Build history of the part. All positions in model axes, mm. Face numbers are marked on the shaded views. A direction names the side the tool comes from. Give positions to 0.01 mm unless a question says otherwise; leave off trailing zeros. Loops run counter-clockwise (first coordinate to the right, second up) from the corner with the lowest first, then second, coordinate; pieces in that order, holes last. Notation, with made-up numbers: (-5.75, -19.75) -> (29.25, -19.75) arc R16 ccw to (29.25, -3.75) -> close; hole circle Ø7 at (34, 81). An arc over 180 degrees is marked (long way). Answer as a JSON object with one key per item and string values. Group by question number.
Q1. Wall check: probe 1 along Y at (x, z) = (15, -64.5); probe 2 along Y at (x, z) = (-15, -63); probe 3 along X at (y, z) = (1.5, 23.5). Give the ranges that are in metal, low to high. Write a range as from..to.
Q2. Band-saw the part on C-C, the plane z = 39. Write the cut outline in (x, y), plus the area to 3 significant figures.
Q3. Tool access for the marked faces 4, 5, 6, 7 and 8: list every direction of +Z, -Z, +X, -X, +Y, -Y with a clear straight run to the whole face (end or side of a thin tool).
Q4. Drop flat-ended pins along their axis: pin 1 (4 mm diameter, centred on y = -21.5, z = 9, fed in from -X); pin 2 (3 mm diameter, centred on x = 11, z = -66.5, fed in from -Y); pin 3 (10 mm diameter, centred on x = 24, y = -38, fed in from -Z). Give the stop position or say it passes through.
Q5. Band-saw the part on D-D, the plane x = -20.5. Write the cut outline in (y, z).
Q6. Band-saw the part on B-B, the plane x = 18. Write the cut outline in (y, z), plus the area to 3 significant figures.
Q7. Band-saw the part on A-A, the plane x = -8. Write the cut outline in (y, z).
Q8. Two-plate mould, pull along Z, no slides. Class the marked faces 1, 2 and 3: pulls with the +Z half, pulls with the -Z half, needs draft (parallel to the pull), parting line crosses it, or undercut.
from build123d import *

# Parameters (mm, degrees)
SKETCH1_R                     = 25
BOSS_EXTRUDE1_DEPTH           = 75
SKETCH2_R                     = 19
BOSS_EXTRUDE2_DEPTH           = 31.75
BOSS_EXTRUDE2_TAPER           = 3
BOSS_EXTRUDE2_OTHER_WAY_DEPTH = 31.75
BOSS_EXTRUDE2_OTHER_WAY_TAPER = 3
CUT_EXTRUDE2_DEPTH            = 161.296002109
CUT_EXTRUDE3_DEPTH            = 161.296002109
SKETCH14_R                    = 12.5
CUT_EXTRUDE4_DEPTH            = 149.240724994
SKETCH16_R                    = 8
CUT_EXTRUDE5_DEPTH            = 159.112302029


with BuildPart() as part:
    # Sketch1 → Boss-Extrude1 (new body)
    with BuildSketch(Plane.XY):
        Circle(SKETCH1_R)
    extrude(amount=BOSS_EXTRUDE1_DEPTH)



with BuildPart() as body_2:
    # Sketch2 → Boss-Extrude2 (new body)
    with BuildSketch(Plane(origin=(0, 0, 0), x_dir=(0, 0, -1), z_dir=(1, 0, 0))):
        with Locations((63.5, -100)):
            Circle(SKETCH2_R)
    extrude(amount=BOSS_EXTRUDE2_DEPTH, taper=BOSS_EXTRUDE2_TAPER)

    # Sketch2 → Boss-Extrude2 other way (add)
    with BuildSketch(Plane(origin=(0, 0, 0), x_dir=(0, 0, -1), z_dir=(1, 0, 0))):
        with Locations((63.5, -100)):
            Circle(SKETCH2_R)
    extrude(amount=-BOSS_EXTRUDE2_OTHER_WAY_DEPTH, taper=BOSS_EXTRUDE2_OTHER_WAY_TAPER)


with BuildPart() as part_1:
    add(part.part)

    add(body_2.part)  # Sweep2 merges body 2
    # Sweep2: sweep along a path in Sketch5
    with BuildLine(Plane(origin=(0, 0, 0), x_dir=(0, 0, -1), z_dir=(1, 0, 0))) as sweep2_path:
        Line((63.5, -81), (8, -81))
        ThreePointArc((8, -81), (-6.142135624, -75.142135624), (-12, -61))
        Line((-12, -61), (-12, 0))
    # Sketch6 → Sweep2 (sweep)
    with BuildSketch(Plane(origin=(0, 0, 0), x_dir=(1, 0, 0), z_dir=(0, 1, 0))):
        Polygon((0, -63.149520499), (-6, -62.835073823), (-6, -28.216088806), (-25, -27.220340999), (-25, -15.220340999), (0, -13.910146517), (25, -15.220340999), (25, -27.220340999), (6, -28.216088806), (6, -62.835073823), align=None)
    sweep(path=sweep2_path.line)

    # Sketch11 → Cut-Extrude2 (cut, through all)
    with BuildSketch(Plane(origin=(6, 0, 0), x_dir=(0, 0, -1), z_dir=(1, 0, 0))):
        with BuildLine():
            Line((63.5, -118.685553324), (-12.864893702, -118.685553324))
            ThreePointArc((-12.864893702, -118.685553324), (-27.962170554, -116.755099832), (-42.087961046, -111.087961046))
            ThreePointArc((-42.087961046, -111.087961046), (-19.107409182, -126.443074889), (8, -131.835073823))
            Line((8, -131.835073823), (63.5, -131.835073823))
            Line((63.5, -131.835073823), (63.5, -118.685553324))
        make_face()
    extrude(amount=-CUT_EXTRUDE2_DEPTH, mode=Mode.SUBTRACT)

    # Sketch13 → Cut-Extrude3 (cut, through all)
    with BuildSketch(Plane(origin=(6, 0, 0), x_dir=(0, 0, -1), z_dir=(1, 0, 0))):
        with BuildLine():
            Line((-45.200625265, -110.295779466), (-42.087961046, -111.087961046))
            ThreePointArc((-42.087961046, -111.087961046), (-36.02411738, -114.035804983), (-29.667824287, -116.28469849))
            Line((-29.667824287, -116.28469849), (-23.461340117, -117.742435424))
            Line((-23.461340117, -117.742435424), (44.847812883, -128.347311627))
            Line((44.847812883, -128.347311627), (71.018240587, -129.970040241))
            Line((71.018240587, -129.970040241), (72.328139591, -135.750206771))
            Line((72.328139591, -135.750206771), (-4.743995253, -135.750206771))
            Line((-4.743995253, -135.750206771), (-39.71664546, -116.755099832))
            Line((-39.71664546, -116.755099832), (-45.200625265, -110.295779466))
        make_face()
    extrude(amount=-CUT_EXTRUDE3_DEPTH, mode=Mode.SUBTRACT)

    # Sketch14 → Cut-Extrude4 (cut, through all)
    with BuildSketch(Plane(origin=(0, 0, 0), x_dir=(-1, 0, 0), z_dir=(0, 0, -1))):
        Circle(SKETCH14_R)
    extrude(amount=-CUT_EXTRUDE4_DEPTH, mode=Mode.SUBTRACT)

    # Sketch16 → Cut-Extrude5 (cut, through all)
    with BuildSketch(Plane.ZY.offset(31.75)):
        with Locations((-63.5, -100)):
            Circle(SKETCH16_R)
    extrude(amount=-CUT_EXTRUDE5_DEPTH, mode=Mode.SUBTRACT)


solid = part_1.part
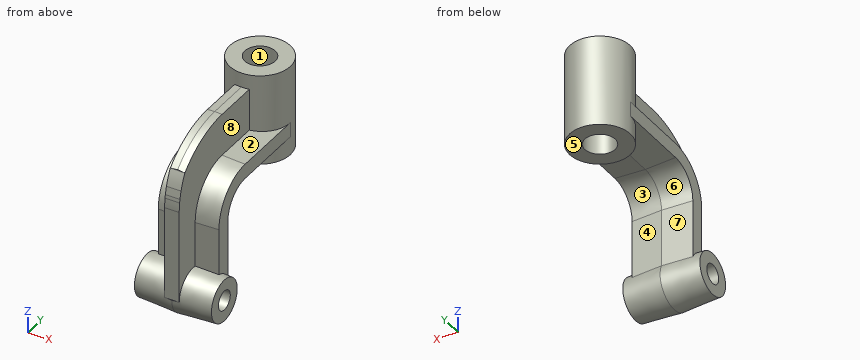
Worked answers:
{
 "1": {"probe 1": "-118.19..-107.94, -92.06..-81.81", "probe 2": "-118.21..-107.98, -92.02..-81.79", "probe 3": "-24.95..-12.41, 12.41..24.95"},
 "2": {"outline": "(-6, -112.69) -> (6, -112.69) -> (6, -24.27) arc R25 ccw (long way) to (-6, -24.27) -> close; hole circle Ø25 at (0, 0)", "area": "2,530 mm2"},
 "3": {"face 4": "+X, +Y", "face 5": "-Z, +X, -X, +Y", "face 6": "-X", "face 7": "-X, +Y", "face 8": "+Z, +X, -Y"},
 "4": {"pin 1": "x = -15.64", "pin 2": "y = -118.38", "pin 3": "z = 14.91"},
 "5": {"outline": "(-96.46, -45.93) arc R17.93 ccw (long way) to (-83.98, -55.45) -> (-83.98, -8) arc R22.98 cw to (-61, 14.98) -> (-14.31, 14.98) -> (-14.31, 0) -> (14.31, 0) -> (14.31, 75) -> (-14.31, 75) -> (-14.31, 27.46) -> (-61, 27.46) arc R35.46 ccw to (-96.46, -8) -> close; hole circle Ø16 at (-100, -63.5)"},
 "6": {"outline": "(-96.59, -45.77) arc R18.06 ccw (long way) to (-83.85, -55.42) -> (-83.85, -8) arc R22.85 cw to (-61, 14.85) -> (-17.35, 14.85) -> (-17.35, 0) -> (17.35, 0) -> (17.35, 75) -> (-17.35, 75) -> (-17.35, 27.59) -> (-61, 27.59) arc R35.59 ccw to (-96.59, -8) -> close; hole circle Ø16 at (-100, -63.5)", "area": "5,090 mm2"},
 "7": {"outline": "(-97.11, -45.15) arc R18.58 ccw (long way) to (-83.33, -55.29) -> (-83.33, -8) arc R22.33 cw to (-61, 14.33) -> (-23.69, 14.33) -> (-23.69, 0) -> (-9.6, 0) -> (-9.6, 75) -> (-23.69, 75) -> (-23.69, 28.11) -> (-61, 28.11) arc R36.11 ccw to (-97.11, -8) -> close; (9.6, 0) -> (23.69, 0) -> (23.69, 75) -> (9.6, 75) -> close; hole circle Ø16 at (-100, -63.5)"},
 "8": {"face 1": "needs draft", "face 2": "pulls with the +Z half", "face 3": "undercut"}
}
